```python
from build123d import *

# Parameters (mm, degrees)
BOSS_EXTRUDE1_DEPTH = 30
CUT_EXTRUDE1_DEPTH  = 2109.570619983


with BuildPart() as part:
    # Sketch1 → Boss-Extrude1 (new body)
    with BuildSketch(Plane.XY):
        Polygon((0, 0), (1015, 0), (1015, 266), (1170, 266), (1170, 1625), (0, 1625), align=None)
    extrude(amount=BOSS_EXTRUDE1_DEPTH)

    # Sketch2 → Cut-Extrude1 (cut, through all)
    with BuildSketch(Plane(origin=(-119.436638294, -43.071405931, 31), x_dir=(1, 0, 0), z_dir=(0, 0, 1))):
        with BuildLine():
            Line((1010.436638294, 1516.071405931), (1010.436638294, 1091.071405931))
            ThreePointArc((1010.436638294, 1091.071405931), (961.230577533, 972.277466691), (842.436638294, 923.071405931))
            Line((842.436638294, 923.071405931), (618.195260429, 923.071405931))
            ThreePointArc((618.195260429, 923.071405931), (516.004262782, 982.071405931), (516.004262782, 1100.071405931))
            Line((516.004262782, 1100.071405931), (790.245640647, 1575.071405931))
            ThreePointArc((790.245640647, 1575.071405931), (922.977285616, 1630.050653433), (1010.436638294, 1516.071405931))
        make_face()
    extrude(amount=-CUT_EXTRUDE1_DEPTH, mode=Mode.SUBTRACT)


solid = part.part
```
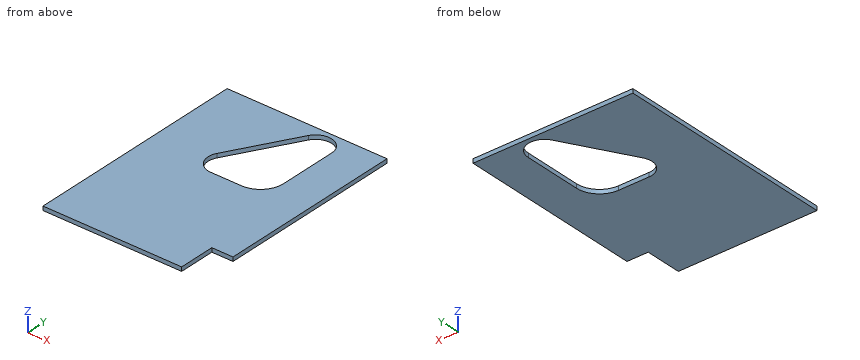
Build history of the part. All positions in model axes, mm. Coordinates: 2 decimals unless noted, no trailing zeros. Order: outer loops, then holes, each group sorted by start corner. A loop starts at its lowest first (then second) coordinate and runs counter-clockwise, first axis right, second up.
Item 1: Drill centre lines: L1, parallel to Y at x = 503, z = 28.25; L2, parallel to Y at x = 1061.5, z = 14.75; L3, parallel to X at y = 1519.5, z = 24. Where is each one in solid material? Low to high.
Filled in:
L1: y = 0 to 880, 1241.35 to 1625
L2: y = 266 to 1625
L3: x = 0 to 663.59, 881.45 to 1170
Item 2: Saw through at C-C on x = 755.5. List the corners of the cut face in (y, z).
Filled in:
outline: (0, 0) - (883.17, 0) - (883.17, 30) - (0, 30) - close; (1589.7, 0) - (1625, 0) - (1625, 30) - (1589.7, 30) - close
Item 3: Saw through at D-D on y = 143.5. List the corners of the cut face in (x, z).
Filled in:
outline: (0, 0) - (1015, 0) - (1015, 30) - (0, 30) - close
Item 4: Saw through at B-B on y = 1156. List the corners of the cut face in (x, z), then the cut area to 3 significant figures.
Filled in:
outline: (0, 0) - (453.73, 0) - (453.73, 30) - (0, 30) - close; (891, 0) - (1170, 0) - (1170, 30) - (891, 30) - close
area: 22,000 mm2
Item 5: Drop flat-ended pins along their axis: pin 1 Ø9 at (x, z) = (1123, 16.5) entering from -Y; pin 2 Ø1.5 at (y, z) = (227.5, 4.5) entering from +X. Give the stop position or say it passes through.
Filled in:
pin 1: stops at y = 266
pin 2: stops at x = 1015
Item 6: Saw through at A-A on z = 17. List the corners of the cut face in (x, y).
Filled in:
outline: (0, 0) - (1015, 0) - (1015, 266) - (1170, 266) - (1170, 1625) - (0, 1625) - close; hole (396.57, 1057) arc R118 ccw to (498.76, 880) - (723, 880) arc R168 ccw to (891, 1048) - (891, 1473) arc R118 ccw to (670.81, 1532) - close
